Build history of the part. All positions in model axes, mm. A direction names the side the tool comes from. Coordinates: 2 decimals unless noted, no trailing zeros. Order: outer loops, then holes, each group sorted by start corner. A loop starts at its lowest first (then second) coordinate and runs counter-clockwise, first axis right, second up. Notation, with made-up numbers: M 71,-10 L 130,-10 A29 ccw 130,14 Z; hole C 12.25,60 d1. An arc over 180 degrees is marked long. Use a Markdown table: item, result. Add a question column.
from build123d import *

# Parameters (mm, degrees)
COPYSKETCH005_R         = 1.8
PAD001_DEPTH            = 1.5
SKETCH005_R             = 3.5
SKETCH005_R_2           = 1.8
PAD002_DEPTH            = 1.5
FILLET_R                = 3.49
SKETCH010_W             = 40
SKETCH010_H             = 11
POCKET005_DEPTH         = 0.4
BODY001_PLACEMENT_ANGLE = 180


with BuildPart() as part:
    # CopySketch005 → Pad001 (new body)
    with BuildSketch(Plane.XY):
        Polygon((-13, -3.9282032303), (-7, -3.9282032303), (-3, 3), (3, 3), (7, -3.9282032303), (13, -3.9282032303), (17, 3), (37.75, 14.5), (37.75, 21.5), (31.75, 21.5), (27.7085481157, 14.5), (-27.7085481157, 14.5), (-31.75, 21.5), (-37.75, 21.5), (-37.75, 14.5), (-17, 3), align=None)
        with Locations((-10, 0)):
            Circle(COPYSKETCH005_R, mode=Mode.SUBTRACT)
        with Locations((10, 0)):
            Circle(COPYSKETCH005_R, mode=Mode.SUBTRACT)
        with Locations((34.25, 18)):
            Circle(COPYSKETCH005_R, mode=Mode.SUBTRACT)
        with Locations((-34.25, 18)):
            Circle(COPYSKETCH005_R, mode=Mode.SUBTRACT)
    extrude(amount=PAD001_DEPTH)

    # Sketch005 (on Face22 of Pad001) → Pad002 (join)
    with BuildSketch(Plane.XY.offset(1.5)):
        with Locations((34.25, 18)):
            Circle(SKETCH005_R)
        with Locations((34.25, 18)):
            Circle(SKETCH005_R_2, mode=Mode.SUBTRACT)
        with Locations((-34.25, 18)):
            Circle(SKETCH005_R)
        with Locations((-34.25, 18)):
            Circle(SKETCH005_R_2, mode=Mode.SUBTRACT)
    extrude(amount=PAD002_DEPTH)

    # Fillet
    fillet_edges = [part.edges().sort_by_distance(p)[0] for p in [
        (-31.75, 21.5, 0.75),
        (-37.75, 21.5, 0.75),
        (-27.708548, 14.5, 0.75),
        (27.708548, 14.5, 0.75),
        (31.75, 21.5, 0.75),
        (37.75, 21.5, 0.75),
        (37.75, 14.5, 0.75),
        (-37.75, 14.5, 0.75),
    ]]
    fillet(fillet_edges, radius=FILLET_R)

    # Sketch010 (on Face30 of Fillet) → Pocket005 (cut)
    with BuildSketch(Plane.XY.offset(1.5)):
        Rectangle(SKETCH010_W, SKETCH010_H)
    extrude(amount=-POCKET005_DEPTH, mode=Mode.SUBTRACT)


with BuildPart() as part_1:
    # Body001 placement: moved
    add(part.part.moved(Location((0, 114.6, 3.6))).rotate(Axis((0, 114.6, 3.6), (0, 1, 0)), BODY001_PLACEMENT_ANGLE))


solid = part_1.part
(1) Drop flat-ended pins along their axis: P1, Ø4.5, axis at x = 34.25, y = 132.6, coming from the -Z side; P2, Ø0.5, axis at x = -4, z = 2.5, coming from the +Y side; P3, Ø3, axis at x = -1.5, y = 117, coming from the -Z side; P4, Ø0.6, axis at x = 0, z = 3, coming from the -Y side. Give the stop position or say it passes through.
(2) Mould opens along Y. For faces 6 (the cylindrical face through (33.419, 131.003, 2.121)), 7 (the flat face through (-29.74, 132.62, 2.86)), 8 (the flat face through (0, 119, 2.5)) say: released by +Y, released by -Y, zero draft, split by the parting line, or undercut.
(3) Slice it at D-D on y = 123.25. Give the cut face in (x, z).
(4) Slice it at B-B on z = 1.4. Give the cut face in (x, y).
(5) Which spindle directions (+Z, -Z, +X, -X, +Y, -Y) get a long thin tool onto all of the face, cutting with end or side? Do faces 1 (the flat face through (-4.972, 114.184, 3.058)), 2 (the cylindrical face through (-33.79, 136.07, 1.36)), 3 (the cylindrical face through (-32.042, 135.645, 2.839)), 4 (the cylindrical face through (-10.831, 113.003, 3.058)), 5 (the cylindrical face through (-37.28, 129.41, 2.84)). Say none if no direction does.
(6) Drill centre lines: line 1 along X through (y, z) = (132.6, 1.55); line 2 along Y through (x, z) = (-10, 3.05); line 3 along X through (y, z) = (114.6, 2.8). Where is each one in solid material? Low to high. Write a range as from..to.
(7) Slice it at A-A on x = -10. Give the cut face in (y, z), and give its area (3 significant figures).
(8) Slice it at C-C on y = 133.25. State how many separate pieces and enclosed holes the cut face has, and give its area (3 significant figures).
Solutions:
| question | item | result |
|---|---|---|
| 1 | P1 | z = 0.6 |
| 1 | P2 | y = 129.1 |
| 1 | P3 | z = 2.5 |
| 1 | P4 | y = 117.6 |
| 2 | face 6 | undercut |
| 2 | face 7 | released by +Y |
| 2 | face 8 | zero draft |
| 3 | outline | M -27.19,2.1 L 27.19,2.1 L 27.19,3.6 L -27.19,3.6 Z |
| 4 | outline | C -34.25,132.6 d7; C 34.25,132.6 d7; hole C -34.25,132.6 d3.6; hole C 34.25,132.6 d3.6 |
| 5 | face 1 | +Z, -Z, -Y |
| 5 | face 2 | -Z |
| 5 | face 3 | +Z, -Z, +Y |
| 5 | face 4 | +Z, -Z |
| 5 | face 5 | +Z, -Z, -X, -Y |
| 6 | line 1 | -37.75..-36.05, -32.45..-30.75, 30.75..32.45, 36.05..37.75 |
| 6 | line 2 | 110.67..112.8, 116.4..129.1 |
| 6 | line 3 | -15.27..-11.8, -8.2..-4.73, 4.73..8.2, 11.8..15.27 |
| 7 | outline | M 110.67,2.5 L 112.8,2.5 L 112.8,3.6 L 110.67,3.6 Z; M 116.4,2.5 L 120.1,2.5 L 120.1,2.1 L 129.1,2.1 L 129.1,3.6 L 116.4,3.6 Z |
| 7 | area | 19.9 mm² |
| 8 | separate pieces | 4 |
| 8 | enclosed holes | 0 |
| 8 | area | 23.3 mm² |
